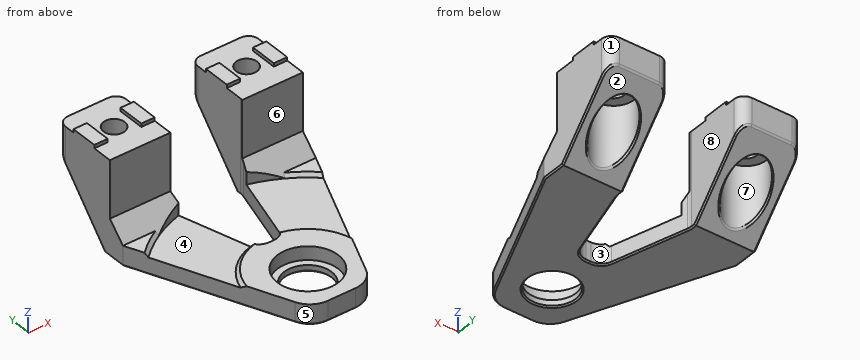
```python
from build123d import *

# Parameters (mm, degrees)
CYLINDER037_R                = 17
CYLINDER037_DEPTH            = 10
CYLINDER036_R                = 38
CYLINDER036_DEPTH            = 10
BOX046_W                     = 4
BOX046_H                     = 8
BOX046_DEPTH                 = 1
BOX045_W                     = 4
BOX045_H                     = 8
BOX045_DEPTH                 = 1
BOX043_W                     = 4
BOX043_H                     = 8
BOX043_DEPTH                 = 1
BOX047_W                     = 4
BOX047_H                     = 8
BOX047_DEPTH                 = 1
CYLINDER033_R                = 3.15
CYLINDER033_DEPTH            = 65
CYLINDER034_R                = 3.15
CYLINDER034_DEPTH            = 65
CYLINDER032_R                = 6.15
CYLINDER032_DEPTH            = 28
CYLINDER031_R                = 6.15
CYLINDER031_DEPTH            = 28
BOX044_W                     = 21.46
BOX044_H                     = 55
BOX044_DEPTH                 = 45
CHAMFER003068012002082_SIZE2 = 7
CHAMFER003068012002082_SIZE  = 25
CHAMFER003068012002083_SIZE2 = 25
CHAMFER003068012002083_SIZE  = 7
FILLET003002010_R            = 4
FILLET003002011_R            = 5
CYLINDER_R                   = 9.05
CYLINDER_DEPTH               = 10
CYLINDER030_R                = 7.05
CYLINDER030_DEPTH            = 10
BOX041_W                     = 57.46
BOX041_H                     = 72
BOX041_DEPTH                 = 6
CHAMFER003068012002084_SIZE2 = 20
CHAMFER003068012002084_SIZE  = 47
CHAMFER003068012002085_SIZE2 = 47
CHAMFER003068012002085_SIZE  = 20
FILLET003002012_R            = 7
BOX042_W                     = 57.46
BOX042_H                     = 20
BOX042_DEPTH                 = 22
CHAMFER003068012002086_SIZE2 = 20
CHAMFER003068012002086_SIZE  = 18
CHAMFER003068012002087_SIZE  = 5
FILLET003002013_R            = 3
CHAMFER003068012002088_SIZE  = 0.99
CHAMFER003068012002089_SIZE  = 0.99
CHAMFER003068012002090_SIZE  = 0.4


with BuildPart() as cylinder037:
    # Cylinder037 → Cylinder037 (new body)
    with BuildSketch(Plane.XY.offset(-23)):
        Circle(CYLINDER037_R)
    extrude(amount=CYLINDER037_DEPTH)


with BuildPart() as cut001040:
    # Cylinder036 → Cylinder036 (new body)
    with BuildSketch(Plane.XY.offset(-23)):
        Circle(CYLINDER036_R)
    extrude(amount=CYLINDER036_DEPTH)

    # Cut001040: cut Cylinder037
    add(cylinder037.part, mode=Mode.SUBTRACT)


with BuildPart() as cube046:
    # Box046 → Box046 (new body)
    with BuildSketch(Plane(origin=(10.73, 45, 0), x_dir=(1, 0, 0), z_dir=(0, 0, 1))):
        with Locations((2, 4)):
            Rectangle(BOX046_W, BOX046_H)
    extrude(amount=BOX046_DEPTH)


with BuildPart() as cube045:
    # Box045 → Box045 (new body)
    with BuildSketch(Plane(origin=(-14.73, 45, 0), x_dir=(1, 0, 0), z_dir=(0, 0, 1))):
        with Locations((2, 4)):
            Rectangle(BOX045_W, BOX045_H)
    extrude(amount=BOX045_DEPTH)


with BuildPart() as cube043:
    # Box043 → Box043 (new body)
    with BuildSketch(Plane(origin=(-28.73, 45, 0), x_dir=(1, 0, 0), z_dir=(0, 0, 1))):
        with Locations((2, 4)):
            Rectangle(BOX043_W, BOX043_H)
    extrude(amount=BOX043_DEPTH)


with BuildPart() as fusion001002012032:
    # Box047 → Box047 (new body)
    with BuildSketch(Plane(origin=(24.73, 45, 0), x_dir=(1, 0, 0), z_dir=(0, 0, 1))):
        with Locations((2, 4)):
            Rectangle(BOX047_W, BOX047_H)
    extrude(amount=BOX047_DEPTH)

    # Fusion001002012032: union Cube046, Cube045, Cube043
    add(cube046.part)
    add(cube045.part)
    add(cube043.part)


with BuildPart() as cylinder033:
    # Cylinder033 → Cylinder033 (new body)
    with BuildSketch(Plane(origin=(-19.73, 49, -41), x_dir=(0, 1, 0), z_dir=(0, 0, 1))):
        Circle(CYLINDER033_R)
    extrude(amount=CYLINDER033_DEPTH)


with BuildPart() as fusion001002012030:
    # Cylinder034 → Cylinder034 (new body)
    with BuildSketch(Plane(origin=(19.73, 49, -41), x_dir=(0, 1, 0), z_dir=(0, 0, 1))):
        Circle(CYLINDER034_R)
    extrude(amount=CYLINDER034_DEPTH)

    # Fusion001002012030: union Cylinder033
    add(cylinder033.part)


with BuildPart() as cylinder032:
    # Cylinder032 → Cylinder032 (new body)
    with BuildSketch(Plane(origin=(-19.73, 49, -41), x_dir=(0, 1, 0), z_dir=(0, 0, 1))):
        Circle(CYLINDER032_R)
    extrude(amount=CYLINDER032_DEPTH)


with BuildPart() as fusion001002012031:
    # Cylinder031 → Cylinder031 (new body)
    with BuildSketch(Plane(origin=(19.73, 49, -41), x_dir=(0, 1, 0), z_dir=(0, 0, 1))):
        Circle(CYLINDER031_R)
    extrude(amount=CYLINDER031_DEPTH)

    # Fusion001002012031: union Cylinder032
    add(cylinder032.part)


with BuildPart() as fusion001002012031_1:
    # Fusion001002012031 placement: moved
    add(fusion001002012031.part.moved(Location((0, 0, 6))))


with BuildPart() as fillet003002011:
    # Box044 → Box044 (new body)
    with BuildSketch(Plane(origin=(-10.73, 14, -35), x_dir=(1, 0, 0), z_dir=(0, 0, 1))):
        with Locations((10.73, 27.5)):
            Rectangle(BOX044_W, BOX044_H)
    extrude(amount=BOX044_DEPTH)

    # Chamfer003068012002082
    chamfer003068012002082_edges = [fillet003002011.edges().sort_by_distance(p)[0] for p in [
        (10.73, 14, -12.5),
    ]]
    chamfer003068012002082_side = fillet003002011.faces().sort_by_distance((10.73, 41.5, -12.5))[0]
    chamfer(chamfer003068012002082_edges, length=CHAMFER003068012002082_SIZE, length2=CHAMFER003068012002082_SIZE2, reference=chamfer003068012002082_side)

    # Chamfer003068012002083
    chamfer003068012002083_edges = [fillet003002011.edges().sort_by_distance(p)[0] for p in [
        (-10.73, 14, -12.5),
    ]]
    chamfer003068012002083_side = fillet003002011.faces().sort_by_distance((-3.5, 14, -12.5))[0]
    chamfer(chamfer003068012002083_edges, length=CHAMFER003068012002083_SIZE, length2=CHAMFER003068012002083_SIZE2, reference=chamfer003068012002083_side)

    # Fillet003002010
    fillet003002010_edges = [fillet003002011.edges().sort_by_distance(p)[0] for p in [
        (-3.73, 14, -12.5),
        (3.73, 14, -12.5),
    ]]
    fillet(fillet003002010_edges, radius=FILLET003002010_R)

    # Fillet003002011
    fillet003002011_edges = [fillet003002011.edges().sort_by_distance(p)[0] for p in [
        (-10.73, 39, -12.5),
        (10.73, 39, -12.5),
    ]]
    fillet(fillet003002011_edges, radius=FILLET003002011_R)


with BuildPart() as cylinder:
    # Cylinder → Cylinder (new body)
    with BuildSketch(Plane.XY.offset(-27)):
        Circle(CYLINDER_R)
    extrude(amount=CYLINDER_DEPTH)


with BuildPart() as fusion001002012028:
    # Cylinder030 → Cylinder030 (new body)
    with BuildSketch(Plane.XY.offset(-29)):
        Circle(CYLINDER030_R)
    extrude(amount=CYLINDER030_DEPTH)

    # Fusion001002012028: union Cylinder
    add(cylinder.part)


with BuildPart() as fusion001002012028_1:
    # Fusion001002012028 placement: moved
    add(fusion001002012028.part.moved(Location((0, 0, 1))))


with BuildPart() as fillet003002012:
    # Box041 → Box041 (new body)
    with BuildSketch(Plane(origin=(-28.73, -13, -28), x_dir=(1, 0, 0), z_dir=(0, 0, 1))):
        with Locations((28.73, 36)):
            Rectangle(BOX041_W, BOX041_H)
    extrude(amount=BOX041_DEPTH)

    # Chamfer003068012002084
    chamfer003068012002084_edges = [fillet003002012.edges().sort_by_distance(p)[0] for p in [
        (-28.73, -13, -25),
    ]]
    chamfer003068012002084_side = fillet003002012.faces().sort_by_distance((-28.73, 23, -25))[0]
    chamfer(chamfer003068012002084_edges, length=CHAMFER003068012002084_SIZE, length2=CHAMFER003068012002084_SIZE2, reference=chamfer003068012002084_side)

    # Chamfer003068012002085
    chamfer003068012002085_edges = [fillet003002012.edges().sort_by_distance(p)[0] for p in [
        (28.73, -13, -25),
    ]]
    chamfer003068012002085_side = fillet003002012.faces().sort_by_distance((10, -13, -25))[0]
    chamfer(chamfer003068012002085_edges, length=CHAMFER003068012002085_SIZE, length2=CHAMFER003068012002085_SIZE2, reference=chamfer003068012002085_side)

    # Fillet003002012
    fillet003002012_edges = [fillet003002012.edges().sort_by_distance(p)[0] for p in [
        (-8.73, -13, -25),
        (8.73, -13, -25),
    ]]
    fillet(fillet003002012_edges, radius=FILLET003002012_R)


with BuildPart() as cut001036:
    # Cut001036 base: copy of Fillet003002012
    add(fillet003002012.part)

    # Cut001036: cut Fusion001002012028
    add(fusion001002012028_1.part, mode=Mode.SUBTRACT)


with BuildPart() as cut001035:
    # Cut001035 base: copy of Fillet003002012
    add(fillet003002012.part)

    # Cut001035: cut Fusion001002012028
    add(fusion001002012028_1.part, mode=Mode.SUBTRACT)


with BuildPart() as obj1:
    # Box042 → Box042 (new body)
    with BuildSketch(Plane(origin=(-28.73, 39, -22), x_dir=(1, 0, 0), z_dir=(0, 0, 1))):
        with Locations((28.73, 10)):
            Rectangle(BOX042_W, BOX042_H)
    extrude(amount=BOX042_DEPTH)

    # Fusion001002012033: union Cut001035
    add(cut001035.part)

    # Fusion001002012034: union Cut001036
    add(cut001036.part)

    # Chamfer003068012002086
    chamfer003068012002086_edges = [obj1.edges().sort_by_distance(p)[0] for p in [
        (0, 59, -28),
    ]]
    chamfer003068012002086_side = obj1.faces().sort_by_distance((0, 30.57213, -28))[0]
    chamfer(chamfer003068012002086_edges, length=CHAMFER003068012002086_SIZE, length2=CHAMFER003068012002086_SIZE2, reference=chamfer003068012002086_side)

    # Cut001037: cut Fillet003002011
    add(fillet003002011.part, mode=Mode.SUBTRACT)

    # Chamfer003068012002087
    chamfer003068012002087_edges = [obj1.edges().sort_by_distance(p)[0] for p in [
        (-19.706303, 39, -22),
        (19.706303, 39, -22),
    ]]
    chamfer(chamfer003068012002087_edges, length=CHAMFER003068012002087_SIZE)

    # Cut001038: cut Fusion001002012031
    add(fusion001002012031_1.part, mode=Mode.SUBTRACT)

    # Cut001039: cut Fusion001002012030
    add(fusion001002012030.part, mode=Mode.SUBTRACT)

    # Fusion001002012035: union Fusion001002012032
    add(fusion001002012032.part)

    # Fillet003002013
    fillet003002013_edges = [obj1.edges().sort_by_distance(p)[0] for p in [
        (-10.73, 59, -4),
        (-28.73, 59, -4),
        (28.73, 59, -4),
        (10.73, 59, -4),
    ]]
    fillet(fillet003002013_edges, radius=FILLET003002013_R)

    # Cut001041: cut Cut001040
    add(cut001040.part, mode=Mode.SUBTRACT)

    # Chamfer003068012002088
    chamfer003068012002088_edges = [obj1.edges().sort_by_distance(p)[0] for p in [
        (11.861461, 12.178085, -22),
        (-11.861461, 12.178085, -22),
    ]]
    chamfer(chamfer003068012002088_edges, length=CHAMFER003068012002088_SIZE)

    # Chamfer003068012002089
    chamfer003068012002089_edges = [obj1.edges().sort_by_distance(p)[0] for p in [
        (-21.735995, 31.169641, -22),
        (21.735995, 31.169641, -22),
    ]]
    chamfer(chamfer003068012002089_edges, length=CHAMFER003068012002089_SIZE)

    # Chamfer003068012002090
    chamfer003068012002090_edges = [obj1.edges().sort_by_distance(p)[0] for p in [
        (-19.636194, 12.629557, -28),
        (-28.73, 48.5, -19.666667),
        (-28.73, 37.5, -28),
        (-7.962252, -11.83893, -28),
        (0, -13, -28),
        (7.962252, -11.83893, -28),
        (19.636194, 12.629557, -28),
        (28.73, 37.5, -28),
        (10.73, 40.343396, -28),
        (10.683489, 39.006389, -28),
        (7.546417, 27.630062, -28),
        (3.11338, 14.812989, -28),
        (0, 14, -28),
        (-3.11338, 14.812989, -28),
        (-7.546417, 27.630062, -28),
        (-10.683489, 39.006389, -28),
        (-10.73, 40.343396, -28),
        (-7.05, 0, -28),
        (-28.042876, 57.910655, -9.210383),
        (-10.73, 48.5, -19.666667),
        (-11.417124, 57.910655, -9.210383),
        (-19.73, 59, -8),
        (-19.723632, 42.850003, -25.944441),
        (28.73, 48.5, -19.666667),
        (10.73, 48.5, -19.666667),
        (28.042876, 57.910655, -9.210383),
        (19.73, 59, -8),
        (11.417124, 57.910655, -9.210383),
        (19.736368, 42.850003, -25.944441),
    ]]
    chamfer(chamfer003068012002090_edges, length=CHAMFER003068012002090_SIZE)


solid = obj1.part
```
Here's how the part is built. I have some questions about the finished solid (model axes, mm). Face numbers are marked on the shaded views. A direction names the side the tool comes from. Give positions to 0.01 mm unless a question says otherwise; leave off trailing zeros. Order: outer loops, then holes, each group sorted by start corner. A loop starts at its lowest first (then second) coordinate and runs counter-clockwise, first axis right, second up. Notation, with made-up numbers: (22, 71.5) -> (32, 71.5) arc R31 cw to (32, 97.5) -> close; hole circle Ø2 at (48, 57.25). An arc over 180 degrees is marked (long way). Use CSV: the item, a comma, the result in double quotes. Start each with the question number.
Item 1: Thinking about a two-plate mould opening in X: for the marked faces 1, 2 and 3, which applies, pulls with the +X half, pulls with the -X half, needs draft (parallel to the pull), parting line crosses it, or undercut?
Item 2: Suppose I cut it at A-A (z = -2). List the corners of the cut face in (x, y) for me, and give its area (3 significant figures).
Item 3: I'm going to push flat-ended pins straight in: P1, Ø1, axis at x = 11.5, z = -8, coming from the +Y side; P2, Ø5, axis at x = -7, z = -7.5, coming from the +Y side; P3, Ø5, axis at x = -21.5, z = -5, coming from the -Y side; P4, Ø10, axis at x = 7, y = 31, coming from the +Z side. Where does each tip first touch, or does it pass through?
Item 4: Suppose I cut it at C-C (y = 49). Give the number of separate pieces and of enclosed holes in the cut face, and give its area (3 significant figures).
Item 5: On a 3-axis mill with a long thin cutter (end or side, diameter ignored), from which of +Z, -Z, +X, -X, +Y, -Y can I reach the whole of each face in a straight line? I mean the marked faces 4, 5, 6, 7 and 8. Say none if no direction works.
Item 6: If I drill on probe 1 along Y at (x, z) = (-19.73, -16.25); probe 2 along Z at (x, y) = (-17.5, 31.5); probe 3 along Y at (x, z) = (-25, -4.25), over which ranges is the centre line in solid material (lowest first)? Write a range as [from, to].
Item 7: Suppose I cut it at B-B (y = 0). List the corners of the cut face in (x, z) for me, and give its area (3 significant figures).
Answer block:
1,face 1,"pulls with the +X half"
1,face 2,"needs draft"
1,face 3,"undercut"
2,outline,"(-28.73, 39) -> (-10.68, 39) arc R5 cw to (-10.73, 39.69) -> (-10.73, 56) arc R3 ccw to (-13.73, 59) -> (-25.73, 59) arc R3 ccw to (-28.73, 56) -> close; (10.68, 39) -> (28.73, 39) -> (28.73, 56) arc R3 ccw to (25.73, 59) -> (13.73, 59) arc R3 ccw to (10.73, 56) -> (10.73, 39.69) arc R5 cw to start; hole circle Ø6.3 at (-19.73, 49); hole circle Ø6.3 at (19.73, 49)"
2,area,"650 mm^2"
3,P1,"stops at y = 58.45"
3,P2,"passes through"
3,P3,"stops at y = 39"
3,P4,"stops at z = -23"
4,separate pieces,"4"
4,enclosed holes,"0"
4,area,"317 mm^2"
5,face 4,"+Z"
5,face 5,"+Z, -Z, -X, -Y"
5,face 6,"+Z, +X, -X, -Y"
5,face 7,"-Z"
5,face 8,"+Z, -Z, +Y"
6,probe 1,"y = [39, 42.85]"
6,probe 2,"z = [-28, -23]"
6,probe 3,"y = [39, 59]"
7,outline,"(-14.26, -27.6) -> (-13.83, -28) -> (-7.45, -28) -> (-7.05, -27.6) -> (-7.05, -26) -> (-9.05, -26) -> (-9.05, -22) -> (-14.26, -22) -> close; (7.05, -27.6) -> (7.45, -28) -> (13.83, -28) -> (14.26, -27.6) -> (14.26, -22) -> (9.05, -22) -> (9.05, -26) -> (7.05, -26) -> close"
7,area,"70.2 mm^2"
